from build123d import *

# Parameters (mm, degrees)
SALIENTE_EXTRUIR1_DEPTH = 100
REDONDEO1_RADIUS        = 50
REDONDEO1_LENGTH        = 20
REDONDEO2_RADIUS        = 50
REDONDEO2_LENGTH        = 20
CROQUIS3_R              = 25
CORTAR_EXTRUIR1_DEPTH   = 174.205080757
CROQUIS10_W             = 20
CROQUIS10_H             = 100
SALIENTE_EXTRUIR3_DEPTH = 100
REDONDEO3_RADIUS        = 50
REDONDEO3_LENGTH        = 20
CROQUIS11_R             = 25
CORTAR_EXTRUIR5_DEPTH   = 154.622914957


with BuildPart() as part:
    # Croquis1 → Saliente-Extruir1 (new body)
    with BuildSketch(Plane(origin=(0, 0, 0), x_dir=(1, 0, 0), z_dir=(0, 1, 0))):
        Polygon((-100, 100), (0, 100), (0, 0), (-100, 0), (-100, 20), (-20, 20), (-20, 80), (-100, 80), align=None)
    extrude(amount=SALIENTE_EXTRUIR1_DEPTH)

    # Redondeo1: full round fillet: the end face becomes a half cylinder, R = half its width
    redondeo1_face = Plane((-100, 50, -90), x_dir=(0, 0, 1), z_dir=(-1, 0, 0))  # on the end face: x along it, z out of the body
    redondeo1_slab = redondeo1_face.offset(-REDONDEO1_RADIUS / 2) * Box(REDONDEO1_LENGTH, 2 * REDONDEO1_RADIUS, REDONDEO1_RADIUS, mode=Mode.PRIVATE)  # the body's end, R deep
    redondeo1_round = Plane((-50, 50, -90), x_dir=(-1, 0, 0), z_dir=(0, 0, 1)) * Cylinder(REDONDEO1_RADIUS, REDONDEO1_LENGTH, mode=Mode.PRIVATE)  # its axis R under the face
    add(redondeo1_slab - redondeo1_round, mode=Mode.SUBTRACT)

    # Redondeo2: full round fillet: the end face becomes a half cylinder, R = half its width
    redondeo2_face = Plane((-100, 50, -10), x_dir=(0, 0, -1), z_dir=(-1, 0, 0))  # on the end face: x along it, z out of the body
    redondeo2_slab = redondeo2_face.offset(-REDONDEO2_RADIUS / 2) * Box(REDONDEO2_LENGTH, 2 * REDONDEO2_RADIUS, REDONDEO2_RADIUS, mode=Mode.PRIVATE)  # the body's end, R deep
    redondeo2_round = Plane((-50, 50, -10), x_dir=(-1, 0, 0), z_dir=(0, 0, -1)) * Cylinder(REDONDEO2_RADIUS, REDONDEO2_LENGTH, mode=Mode.PRIVATE)  # its axis R under the face
    add(redondeo2_slab - redondeo2_round, mode=Mode.SUBTRACT)

    # Croquis3 → Cortar-Extruir1 (cut, through all)
    with BuildSketch(Plane.XY):
        with Locations((-50, 50)):
            Circle(CROQUIS3_R)
    extrude(amount=-CORTAR_EXTRUIR1_DEPTH, mode=Mode.SUBTRACT)

    # Croquis10 → Saliente-Extruir3 (add)
    with BuildSketch(Plane(origin=(0, 0, 0), x_dir=(0, 0, -1), z_dir=(1, 0, 0))):
        with Locations((50, 50)):
            Rectangle(CROQUIS10_W, CROQUIS10_H)
    extrude(amount=SALIENTE_EXTRUIR3_DEPTH)

    # Redondeo3: full round fillet: the end face becomes a half cylinder, R = half its width
    redondeo3_face = Plane((100, 50, -50), x_dir=(0, 0, 1), z_dir=(1, 0, 0))  # on the end face: x along it, z out of the body
    redondeo3_slab = redondeo3_face.offset(-REDONDEO3_RADIUS / 2) * Box(REDONDEO3_LENGTH, 2 * REDONDEO3_RADIUS, REDONDEO3_RADIUS, mode=Mode.PRIVATE)  # the body's end, R deep
    redondeo3_round = Plane((50, 50, -50), x_dir=(1, 0, 0), z_dir=(0, 0, 1)) * Cylinder(REDONDEO3_RADIUS, REDONDEO3_LENGTH, mode=Mode.PRIVATE)  # its axis R under the face
    add(redondeo3_slab - redondeo3_round, mode=Mode.SUBTRACT)

    # Croquis11 → Cortar-Extruir5 (cut, through all)
    with BuildSketch(Plane.XY.offset(-40)):
        with Locations((50, 50)):
            Circle(CROQUIS11_R)
    extrude(amount=-CORTAR_EXTRUIR5_DEPTH, mode=Mode.SUBTRACT)


solid = part.part
Can you work these out from the model? Positions are in its coordinate system, mm. A direction names the side the tool comes from. Coordinates: 2 decimals unless noted, no trailing zeros. Order: outer loops, then holes, each group sorted by start corner. A loop starts at its lowest first (then second) coordinate and runs counter-clockwise, first axis right, second up. Notation, with made-up numbers: M -21.5,-38.75 L 31.5,-38.75 A15 ccw 31.5,-34.75 Z; hole C 12,-37.5 d9. An arc over 180 degrees is marked long. Answer as CSV lines item,"result".
(1) Please list where these lines run through material, in increasing order: L1, parallel to Z at x = -23.5, y = 44; L2, parallel to Z at x = 13, y = 92; L3, parallel to Y at x = 50, z = -55.5.
Geometry check:
L1,"-100 to -80, -20 to 0"
L2,"-60 to -40"
L3,"0 to 25, 75 to 100"
(2) On a 3-axis mill with a long thin cutter (end or side, diameter ignored), from which of +Z, -Z, +X, -X, +Y, -Y can I reach the whole of each face in a straight line? I mean faces 5 (the flat face through (27, 38, -40)), 6 (the flat face through (-77, 49, -80)), 7 (the flat face through (0, 49, -80)). Say none if no direction works.
Geometry check:
face 5,"+Z, +X, +Y, -Y"
face 6,"-X, +Y, -Y"
face 7,"-Z, +X, +Y, -Y"
(3) Suppose I cut it at A-A on y = 50. Please give me the cut outline in (x, z), plus the area to 3 significant figures.
Geometry check:
outline,"M -100,-100 L -75,-100 L -75,-80 L -100,-80 Z; M -100,-20 L -75,-20 L -75,0 L -100,0 Z; M -25,-100 L 0,-100 L 0,-60 L 25,-60 L 25,-40 L 0,-40 L 0,0 L -25,0 L -25,-20 L -20,-20 L -20,-80 L -25,-80 Z; M 75,-60 L 100,-60 L 100,-40 L 75,-40 Z"
area,"4,200 mm^2"
(4) I'm going to push flat-ended pins straight in: pin 1 (12 mm diameter, centred on y = 48.5, z = -28.5, fed in from +X); pin 2 (12 mm diameter, centred on y = 88, z = -49.5, fed in from -X); pin 3 (4 mm diameter, centred on x = 38, y = 72, fed in from -Z). Where does each tip first touch, or does it pass through?
Geometry check:
pin 1,"x = 0"
pin 2,"x = -20"
pin 3,"z = -60"
(5) Suppose I cut it at B-B on x = -73. Please give me the cut outline in (y, z), plus the area to 3 significant figures.
Geometry check:
outline,"M 5.6,-100 L 40.2,-100 L 40.2,-80 L 5.6,-80 Z; M 5.6,-20 L 40.2,-20 L 40.2,0 L 5.6,0 Z; M 59.8,-100 L 94.4,-100 L 94.4,-80 L 59.8,-80 Z; M 59.8,-20 L 94.4,-20 L 94.4,0 L 59.8,0 Z"
area,"2,770 mm^2"
(6) If we mould it in two halves opening along Y, with no side actions, what happens to faces 1 (the flat face through (-11, 0, -50)), 2 (the flat face through (0, 49, -20)), 3 (the flat face through (-11, 100, -50)), 4 (the cylindrical face through (-70, 35, -90))? For each: released by +Y, released by -Y, zero draft, split by the parting line, or undercut.
Geometry check:
face 1,"released by -Y"
face 2,"zero draft"
face 3,"released by +Y"
face 4,"undercut"
(7) Suppose I cut it at C-C on z = -43. Please give me the cut outline in (x, y), plus the area to 3 significant figures.
Geometry check:
outline,"M -20,0 L 50,0 A50 ccw 50,100 L -20,100 Z; hole C 50,50 d50"
area,"8,960 mm^2"
(8) Suppose I cut it at D-D on y = 17. Please give me the cut outline in (x, z).
Geometry check:
outline,"M -87.56,-100 L 0,-100 L 0,-60 L 87.56,-60 L 87.56,-40 L 0,-40 L 0,0 L -87.56,0 L -87.56,-20 L -20,-20 L -20,-80 L -87.56,-80 Z"
